```python
from build123d import *

# Parameters (mm, degrees)
SKICA2_R                 = 3.5
ODEBRAT_VYSUNUT_M1_DEPTH = 6
KRUHOV_POLE1_COUNT       = 4
ZAOBLIT1_R               = 3
ZAOBLIT2_R               = 1
ZAOBLIT3_R               = 5


with BuildPart() as part:
    # Skica1 → Rotovat1 (revolve)
    with BuildSketch(Plane(origin=(0, 0, 0), x_dir=(0, 0, -1), z_dir=(1, 0, 0))):
        Polygon((0, 64), (0, 0), (6, 0), (6, 29), (16, 29), (16, 34), (6, 34), (6, 64), align=None)
    revolve(axis=Axis((0, 0, 30.782343988), (0, 0, -1)))

    # Skica2 → Odebrat vysunutím1 (cut)
    with BuildSketch(Plane.XY):
        with Locations((0, 50)):
            Circle(SKICA2_R)
    odebrat_vysunut_m1 = extrude(amount=-ODEBRAT_VYSUNUT_M1_DEPTH, mode=Mode.SUBTRACT)

    # Kruhové pole1: Odebrat vysunutím1 ×4 about axis
    kruhov_pole1_axis = Axis((0, -0.149984695, 0), (0, 0, 1))
    for i in range(1, KRUHOV_POLE1_COUNT):
        add(odebrat_vysunut_m1.rotate(kruhov_pole1_axis, i * 360 / KRUHOV_POLE1_COUNT), mode=Mode.SUBTRACT)

    # Zaoblit1
    zaoblit1_edges = [part.edges().sort_by_distance(p)[0] for p in [
        (0, -64, 0),
    ]]
    fillet(zaoblit1_edges, radius=ZAOBLIT1_R)

    # Zaoblit2
    zaoblit2_edges = [part.edges().sort_by_distance(p)[0] for p in [
        (0, -34, -6),
    ]]
    fillet(zaoblit2_edges, radius=ZAOBLIT2_R)

    # Zaoblit3
    zaoblit3_edges = [part.edges().sort_by_distance(p)[0] for p in [
        (0, -29, -6),
    ]]
    fillet(zaoblit3_edges, radius=ZAOBLIT3_R)


solid = part.part
```
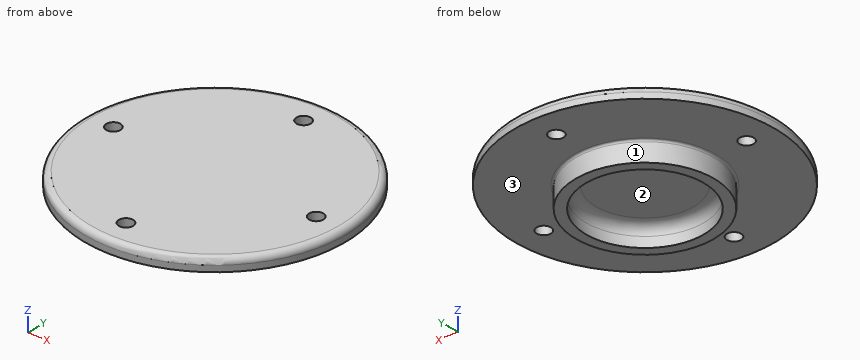
Geometry: final body of the model. Coordinates: model frame, mm. Face numbers are marked on the shaded views. Round coordinates to 2 decimals unless told otherwise and drop trailing zeros. Order: outer loops, then holes, each group sorted by start corner. A loop starts at its lowest first (then second) coordinate and runs counter-clockwise, first axis right, second up. Notation, with made-up numbers: (82.25, -14.5) - (93.25, -14.5) arc R20 ccw to (93.25, 10.5) - close; hole circle Ø8 at (2.25, 54.25). An arc over 180 degrees is marked (long way). Write item = value, one per line. Start each with the question number.
Q1. Pin query (flat end, axial travel): pin 1 (1.5 mm diameter, centred on x = 51, y = -26, fed in from -Z); pin 2 (3 mm diameter, centred on x = -44.5, y = 11.5, fed in from +Z); pin 3 (1 mm diameter, centred on x = -22, z = -11.5, fed in from +Y); pin 4 (5 mm diameter, centred on y = 17, z = -4.5, fed in from +X). Return the tip coordinate at first contact, or that it passes through.
Q2. Ray query, line 1 (X direction, y = 0, z = -14.65); line 2 (Z direction, x = 44, y = -31); line 3 (X direction, y = -17, z = -7.75). Return the intervals inside material, ascending. Write a range as from..to.
Q3. Pull-direction query (X, two-part tool) for the marked faces 1, 2 and 3; classes: +X half, -X half, draft (parallel to the pull), parting line (faces both ways), or undercut.
Q4. Cut plane C-C on z = -1.5. Return the cut outline in (x, y), and give its area (3 significant figures).
Q5. Cut plane A-A on x = 0. Return the cut outline in (y, z), and give its area (3 significant figures).
Q6. Cut plane B-B on y = 0. Return the cut outline in (x, z).
Q7. Cut plane D-D on z = -9.25. Return the cut outline in (x, y).
Outcome:
q1.pin_1 = -6
q1.pin_2 = 0
q1.pin_3 = 26.34
q1.pin_4 = 62.34
q2.line_1 = -34..-29, 29..34
q2.line_2 = -6..0
q2.line_3 = -29.44..-22, 22..29.44
q3.face_1 = parting line
q3.face_2 = undercut
q3.face_3 = draft
q4.outline = circle Ø127.2 at (0, 0); hole circle Ø7 at (-50.15, -0.15); hole circle Ø7 at (0, -50.3); hole circle Ø7 at (0, 50); hole circle Ø7 at (50.15, -0.15)
q4.area = 12,600 mm^2
q5.outline = (-64, -6) - (-53.8, -6) - (-53.8, 0) - (-61, 0) arc R3 ccw to (-64, -3) - close; (-46.8, -6) - (-35, -6) arc R1 cw to (-34, -7) - (-34, -16) - (-29, -16) - (-29, -11) arc R5 cw to (-24, -6) - (24, -6) arc R5 cw to (29, -11) - (29, -16) - (34, -16) - (34, -7) arc R1 cw to (35, -6) - (46.5, -6) - (46.5, 0) - (-46.8, 0) - close; (53.5, -6) - (64, -6) - (64, -3) arc R3 ccw to (61, 0) - (53.5, 0) - close
q5.area = 791 mm^2
q6.outline = (-64, -6) - (-53.65, -6) - (-53.65, 0) - (-61, 0) arc R3 ccw to (-64, -3) - close; (-46.65, -6) - (-35, -6) arc R1 cw to (-34, -7) - (-34, -16) - (-29, -16) - (-29, -11) arc R5 cw to (-24, -6) - (24, -6) arc R5 cw to (29, -11) - (29, -16) - (34, -16) - (34, -7) arc R1 cw to (35, -6) - (46.65, -6) - (46.65, 0) - (-46.65, 0) - close; (53.65, -6) - (64, -6) - (64, -3) arc R3 ccw to (61, 0) - (53.65, 0) - close
q7.outline = circle Ø68 at (0, 0); hole circle Ø57.37 at (0, 0)
